```python
from build123d import *

# Parameters (mm, degrees)
SKETCH1_R           = 12.1
BOSS_EXTRUDE1_DEPTH = 30.5
SKETCH2_R           = 3.175
BOSS_EXTRUDE2_DEPTH = 1.6
SKETCH3_R           = 1
BOSS_EXTRUDE3_DEPTH = 10.4
SKETCH4_R           = 4.25
BOSS_EXTRUDE4_DEPTH = 2
FILLET1_R           = 1
FILLET2_R           = 0.5


with BuildPart() as part:
    # Sketch1 → Boss-Extrude1 (new body)
    with BuildSketch(Plane.XY):
        with Locations(Location((0, 0, 0), (0, 0, 180))):
            Circle(SKETCH1_R)
    extrude(amount=BOSS_EXTRUDE1_DEPTH)

    # Sketch2 → Boss-Extrude2 (add)
    with BuildSketch(Plane.XY.offset(30.5)):
        Circle(SKETCH2_R)
    extrude(amount=BOSS_EXTRUDE2_DEPTH)

    # Sketch3 → Boss-Extrude3 (add)
    with BuildSketch(Plane.XY.offset(32.1)):
        Circle(SKETCH3_R)
    extrude(amount=BOSS_EXTRUDE3_DEPTH)

    # Sketch4 → Boss-Extrude4 (add)
    with BuildSketch(Plane(origin=(0, 0, 0), x_dir=(-1, 0, 0), z_dir=(0, 0, -1))):
        with Locations(Location((0, 0, 0), (0, 0, 180))):
            Circle(SKETCH4_R)
    extrude(amount=BOSS_EXTRUDE4_DEPTH)

    # Fillet1
    fillet1_edges = [part.edges().sort_by_distance(p)[0] for p in [
        (12.1, 0, 0),
        (12.1, 0, 30.5),
    ]]
    fillet(fillet1_edges, radius=FILLET1_R)

    # Fillet2
    fillet2_edges = [part.edges().sort_by_distance(p)[0] for p in [
        (-4.25, 0, -2),
        (-3.175, 0, 32.1),
    ]]
    fillet(fillet2_edges, radius=FILLET2_R)


solid = part.part
```
Work out the finished part from the listing and answer in its coordinate system (mm). A direction names the side the tool comes from. Coordinates: 2 decimals unless noted, no trailing zeros. Loops run counter-clockwise (first coordinate to the right, second up) from the corner with the lowest first, then second, coordinate; pieces in that order, holes last. Notation, with made-up numbers: (80.25, 48.5) -> (120.25, 48.5) arc R21 ccw to (120.25, 85.5) -> close; hole circle Ø8 at (6.5, 7.5). An arc over 180 degrees is marked (long way). Answer as CSV lines item,"result".
Q1. The part is cut by section C-C on z = 19.5. Write down the section's boundary in (x, y), and give its area (3 significant figures).
Findings:
outline,"circle Ø24.2 at (0, 0)"
area,"460 mm²"
Q2. Each of these flat-tipped pins is pushed along its axis until it touches: pin 1 (10 mm diameter, centred on x = 0, z = 34, fed in from -Y); pin 2 (6 mm diameter, centred on x = 8, y = -2, fed in from +Z); pin 3 (8 mm diameter, centred on y = -6, z = 30, fed in from +X); pin 4 (6 mm diameter, centred on x = 3, z = 31.5, fed in from +Y). Where does it stop, or does it pass through?
Findings:
pin 1,"stops at y = -12.1"
pin 2,"stops at z = 30.5"
pin 3,"stops at x = 11.93"
pin 4,"stops at y = 12.08"
Q3. A tool of negligible diameter and unlimited length cuts with its end or side. For faces 1 (the face through (0, 0, -2)), 2 (the face through (-5, 0, 0)), 3 (the face through (0, -1, 37)), from which of +Z, -Z, +X, -X, +Y, -Y can it reach the whole face along a straight path? Write none if from no direction.
Findings:
face 1,"-Z, +X, -X, +Y, -Y"
face 2,"-Z"
face 3,"+Z"
Q4. Find the intervals of material crossed by probe 1 along Z at (x, y) = (1, -4.25); probe 2 along Z at (x, y) = (0.5, -2.5); probe 3 along X at (y, z) = (6.5, 17.5), in increasing order.
Findings:
probe 1,"z = 0 to 30.5"
probe 2,"z = -2 to 32.1"
probe 3,"x = -10.21 to 10.21"
Q5. The part is cut by section A-A on y = 0. Write down the section's boundary in (x, z) (3 decimals), and give its area (3 significant figures).
Findings:
outline,"(-12.1, 1) arc R1 ccw to (-11.1, 0) -> (-4.25, 0) -> (-4.25, -1.5) arc R0.5 ccw to (-3.75, -2) -> (3.75, -2) arc R0.5 ccw to (4.25, -1.5) -> (4.25, 0) -> (11.1, 0) arc R1 ccw to (12.1, 1) -> (12.1, 29.5) arc R1 ccw to (11.1, 30.5) -> (3.175, 30.5) -> (3.175, 31.6) arc R0.5 ccw to (2.675, 32.1) -> (1, 32.1) -> (1, 42.5) -> (-1, 42.5) -> (-1, 32.1) -> (-2.675, 32.1) arc R0.5 ccw to (-3.175, 31.6) -> (-3.175, 30.5) -> (-11.1, 30.5) arc R1 ccw to (-12.1, 29.5) -> close"
area,"785 mm²"
